Source: CAD feature listing. Evaluate the final solid. Frame: model axes, mm. Face numbers are marked on the shaded views. Coordinates: 2 decimals unless noted, no trailing zeros. Order: outer loops, then holes, each group sorted by start corner. A loop starts at its lowest first (then second) coordinate and runs counter-clockwise, first axis right, second up. Notation, with made-up numbers: (22.5, 62.25) -> (39.5, 62.25) arc R29 cw to (39.5, 91.25) -> close; hole circle Ø6 at (89, -39.75). An arc over 180 degrees is marked (long way). Put each result on its own line as item: value.
Autodesk Inventor part; units mm, degrees
ref_plane "YZ Plane" through (0, 0, 0) normal (1, 0, 0) x (0, 1, 0)
ref_plane "XZ Plane" through (0, 0, 0) normal (0, 1, 0) x (-1, 0, 0)
ref_plane "XY Plane" through (0, 0, 0) normal (0, 0, 1) x (1, 0, 0)
sketch "Sketch1" plane through (0, 0, 0) normal (0, 0, 1) x (1, 0, 0)
  line L0 (-36, -250) -> (36, -250)
  line L1 (36, -250) -> (36, 250)
  line L2 (36, 250) -> (-36, 250)
  line L3 (-36, 250) -> (-36, -250)
  line L4 (-36, -250) -> (36, 250) construction
  line L5 (36, -250) -> (-36, 250) construction
  point P0 (0, 0)
  dimension "d154" = 72
  dimension "d155" = 500
extrude "Plate5" add sketch "Sketch1" along normal blind 2
sketch "Sketch7" plane through (-34, -250, 0) normal (-1, 0, 0) x (0, -1, 0)
  line L0 (-500, 0) -> (0, 0)
  line L1 (0, 0) -> (0, 64)
  line L2 (0, 64) -> (-500, 64)
  line L3 (-500, 64) -> (-500, 0)
edge flange "Flange3" height 64 angle 90 thickness 2 bend radius 2.75 thickness toward (-1, 0, 0) relief round relief width 2 relief depth 1 edges at (-36, 0, 2) wall of the first edge with corners at (-34, 250, 0) (-34, -250, 0) (-34, -250, 64) (-34, 250, 64)
bend "Bend3"
corner "Corner3"
properties part number "PNS 753 FDS 1200 FLANGE 3" material "Stainless Steel"
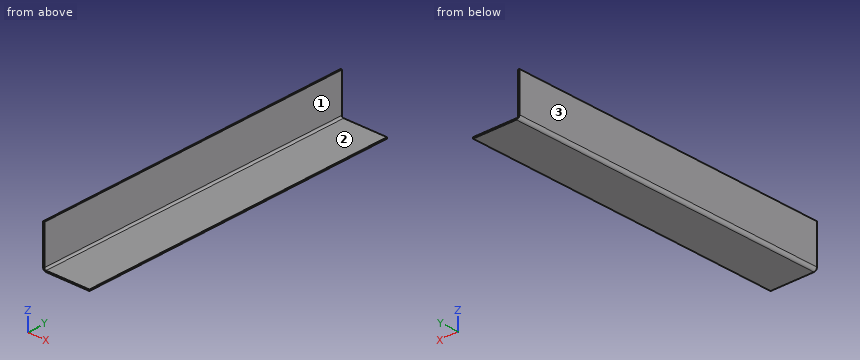
1. Cut plane A-A on y = -48.5. Output: boundary loops of the cut face in (x, z), plus the area to 3 significant figures.
Numbers:
outline: (-36, 4.75) arc R4.75 ccw to (-31.25, 0) -> (36, 0) -> (36, 2) -> (-31.25, 2) arc R2.75 cw to (-34, 4.75) -> (-34, 64) -> (-36, 64) -> close
area: 265 mm2
2. Cut plane C-C on z = 53.5. Output: boundary loops of the cut face in (x, y).
Numbers:
outline: (-36, -250) -> (-34, -250) -> (-34, 250) -> (-36, 250) -> close
3. Ray query, line 1 along Z through (x, y) = (3, -110); line 2 along X through (y, z) = (-223, 34). Return the intervals inside material, ascending.
Numbers:
line 1: z = 0 to 2
line 2: x = -36 to -34
4. Cut plane B-B on x = -16. Output: boundary loops of the cut face in (y, z).
Numbers:
outline: (-250, 0) -> (250, 0) -> (250, 2) -> (-250, 2) -> close
5. Pull-direction query (X, two-part tool) for the marked faces 1, 2 and 3; classes: pulls with the +X half, pulls with the -X half, needs draft (parallel to the pull), parting line crosses it, or undercut.
Numbers:
face 1: pulls with the +X half
face 2: needs draft
face 3: pulls with the -X half
6. First-contact query: pin 1 (5 mm diameter, centred on x = 25.5, y = -153.5, fed in from +Z); pin 2 (18 mm diameter, centred on y = -23.5, z = 30, fed in from +X). Flat tips, straight axial feed; report the tip coordinate or a pass-through.
Numbers:
pin 1: stops at z = 2
pin 2: stops at x = -34
